Verification items for the finished model (mm, model axes). A direction names the side the tool comes from. Coordinates: 2 decimals unless noted, no trailing zeros. Write each loop counter-clockwise with the first axis right and the second up, starting at its lowest first coordinate (ties: lowest second). Pieces come first, ordered by that corner, then holes. Notation, with made-up numbers: (67.5, 47) -> (92.5, 47) arc R25 ccw to (92.5, 64) -> close; hole circle Ø9 at (43, 48.25). An arc over 180 degrees is marked (long way). Use CSV: the item, a comma, the result in double quotes.
Autodesk Inventor part; units mm, degrees
ref_plane "YZ Plane" through (0, 0, 0) normal (1, 0, 0) x (0, 1, 0)
ref_plane "XZ Plane" through (0, 0, 0) normal (0, 1, 0) x (-1, 0, 0)
ref_plane "XY Plane" through (0, 0, 0) normal (0, 0, 1) x (1, 0, 0)
sketch "Náčrt1" plane through (0, 0, 0) normal (0, 0, 1) x (1, 0, 0)
  line L0 (-9, 0) -> (-5, 0)
  line L1 (-5, 0) -> (-5, 7)
  line L2 (-5, 7) -> (5, 7)
  line L3 (5, 7) -> (5, 0)
  line L4 (9, 0) -> (9, 15)
  line L5 (9, 15) -> (-9, 15)
  line L6 (-9, 15) -> (-9, 0)
  line L7 (5, 0) -> (9, 0)
  point P0 (0, 0)
  dimension "d0" = 10
  dimension "d1" = 4
  dimension "d2" = 4
  dimension "d3" = 5
  dimension "d4" = 7
  dimension "d5" = 7
  dimension "d8" = 8
extrude "Vysunutí1" add sketch "Náčrt1" along normal blind 10
sketch "Náčrt2" plane through (0, 0, 0) normal (0, 0, -1) x (-1, 0, 0)
  line L0 (5, 7) -> (-5, 7)
  line L1 (-12, 15) -> (12, 15)
  line L2 (12, 15) -> (12, 8.5)
  line L3 (12, 8.5) -> (-12, 8.5)
  line L4 (-12, 8.5) -> (-12, 15)
  line L5 (-9, 15) -> (9, 15)
  line L6 (-9, 0) -> (-9, 15)
  line L7 (9, 15) -> (9, 0)
  point P0 (0, 0)
  dimension "d19" = 1.5
  dimension "d20" = 3
  dimension "d21" = 3
extrude "Vysunutí4" add sketch "Náčrt2" along normal blind 15
sketch "Náčrt4" plane through (-9, 15, 10) normal (0, 1, 0) x (1, 0, 0)
  line L0 (21, 25) -> (-3, 25)
  line L1 (1.9, 25) -> (16.1, 25)
  line L2 (16.1, 25) -> (16.1, 13)
  line L3 (16.1, 13) -> (1.9, 13)
  line L4 (1.9, 13) -> (1.9, 25)
  line L5 (21, 10) -> (21, 25)
  line L6 (-3, 10) -> (-3, 25)
  point P0 (9, 10)
  dimension "d24" = 12
  dimension "d25" = 4.9
  dimension "d26" = 4.9
extrude "Vysunutí5" cut sketch "Náčrt4" against normal blind 15
sketch "Náčrt5" plane through (0, 0, -15) normal (0, 0, -1) x (-1, 0, 0)
  line L0 (-7.1, 15) -> (-12, 15)
  line L1 (12, 8.5) -> (12, 15)
  line L2 (-12, 15) -> (12, 15)
  line L3 (12, 15) -> (12, 8.5)
  line L4 (12, 8.5) -> (-12, 8.5)
  line L5 (-12, 8.5) -> (-12, 15)
  point P0 (0, 0)
extrude "Vysunutí6" add sketch "Náčrt5" along normal blind 10
sketch "Náčrt6" plane through (-9, 15, 10) normal (0, 1, 0) x (1, 0, 0)
  line L0 (2, 28) -> (6, 28)
  line L1 (6, 28) -> (6, 33)
  line L2 (6, 33) -> (2, 33)
  line L3 (2, 33) -> (2, 28)
  line L4 (12, 28) -> (16, 28)
  line L5 (16, 28) -> (16, 33)
  line L6 (16, 33) -> (12, 33)
  line L7 (12, 33) -> (12, 28)
  line L8 (-3, 10) -> (-3, 35)
  line L9 (21, 10) -> (21, 35)
  line L10 (1.9, 25) -> (16.1, 25)
  line L11 (-3, 35) -> (21, 35)
  point P0 (9, 10)
  dimension "d33" = 3
  dimension "d34" = 3
  dimension "d35" = 2
  dimension "d36" = 2
  dimension "d38" = 4
  dimension "d39" = 4
  dimension "d45" = 6
  dimension "d46" = 5
  dimension "d47" = 5
extrude "Vysunutí7" cut sketch "Náčrt6" against normal blind 10
fillet "Zaoblení2" radius 1.2 10 edges at (-9, 7.5, 10) (-9, 4.25, 0) (9, 4.25, 0) (9, 7.5, 10) (9, 11.75, 0) (12, 11.75, 0) (-9, 11.75, 0) (-12, 11.75, 0) (-12, 11.75, -25) (12, 11.75, -25)
equation "\"d2\" = d1"
equation "\"d5\" = d4"
equation "\"d21\" = d20"
equation "\"d26\" = d25"
equation "\"d34\" = d33"
equation "\"d36\" = d35"
equation "\"d39\" = d38"
properties part number "QRholder-bottom"
1) Gauge pin test, flat ends, axial feed: pin 1 (5.5 mm diameter, centred on y = 2, z = 4.5, fed in from -X); pin 2 (4 mm diameter, centred on y = 10.5, z = 4, fed in from +X). Record the tip position at first contact, or that the pin passes through.
Return value:
pin 1,"x = -9"
pin 2,"x = 9"
2) Cross-section at A-A (z = -22). Record the boundary of the cut face in (x, y).
Return value:
outline,"(-12, 8.5) -> (-7, 8.5) -> (-7, 15) -> (-12, 15) -> close; (-3, 8.5) -> (3, 8.5) -> (3, 15) -> (-3, 15) -> close; (7, 8.5) -> (12, 8.5) -> (12, 15) -> (7, 15) -> close"
3) Set-up check for faces 4 (the flat face through (7, 0, 5)), 5 (the flat face through (-9, 8, 5)), 6 (the flat face through (7.1, 12, -9)), 7 (the flat face through (-5, 3, 5)), 8 (the cylindrical face through (8.658, 4.31, 0.361)): record each of +Z, -Z, +X, -X, +Y, -Y from which the full face is reachable in a straight line by a thin tool's end or side.
Return value:
face 4,"+Z, -Z, +X, -X, -Y"
face 5,"+Z, -X, +Y, -Y"
face 6,"+Y, -Y"
face 7,"+Z, -Z, -Y"
face 8,"-Z, +X, -Y"
4) Cross-section at D-D (z = -12.5). Record the boundary of the cut face in (x, y), plus the area to 3 significant figures.
Return value:
outline,"(-12, 8.5) -> (-7.1, 8.5) -> (-7.1, 15) -> (-12, 15) -> close; (7.1, 8.5) -> (12, 8.5) -> (12, 15) -> (7.1, 15) -> close"
area,"63.7 mm2"
5) Cross-section at B-B (y = 6.25). Record the boundary of the cut face in (x, z), plus the area to 3 significant figures.
Return value:
outline,"(-9, 1.2) arc R1.2 ccw to (-7.8, 0) -> (-5, 0) -> (-5, 10) -> (-7.8, 10) arc R1.2 ccw to (-9, 8.8) -> close; (5, 0) -> (7.8, 0) arc R1.2 ccw to (9, 1.2) -> (9, 8.8) arc R1.2 ccw to (7.8, 10) -> (5, 10) -> close"
area,"78.8 mm2"
6) Cross-section at C-C (x = -6.25). Record the boundary of the cut face in (y, z).
Return value:
outline,"(0, 0) -> (8.5, 0) -> (8.5, -3) -> (15, -3) -> (15, 10) -> (0, 10) -> close; (8.5, -25) -> (15, -25) -> (15, -23) -> (8.5, -23) -> close; (8.5, -18) -> (15, -18) -> (15, -15) -> (8.5, -15) -> close"
7) Mould release check, pull along Z, two halves, no side actions. Record for faces 1 (the flat face through (-7.1, 12, -9)), 2 (the flat face through (-7, 0, 5)), 3 (the flat face through (0, 9, 10)): released by +Z, released by -Z, zero draft, split by the parting line, or undercut.
Return value:
face 1,"undercut"
face 2,"zero draft"
face 3,"released by +Z"
8) Scan lines: L1, parallel to Z at x = 6.25, y = 11.75; L2, parallel to X at y = 4.25, z = 3; L3, parallel to X at y = 11, z = -6. Record each from-to range of solid material in increasing order.
Return value:
L1,"-25 to -23, -18 to -15, -3 to 10"
L2,"-9 to -5, 5 to 9"
L3,"-12 to -7.1, 7.1 to 12"
